```python
from build123d import *

# Parameters (mm, degrees)
SKETCH1_W               = 41.75
SKETCH1_H               = 14
BOSS_EXTRUDE1_DEPTH     = 6.5
SKETCH2_W               = 18
SKETCH2_H               = 14
BOSS_EXTRUDE2_DEPTH     = 26.8
CUT_EXTRUDE1_DEPTH      = 56.20826478
CUT_EXTRUDE1_DEPTH_BACK = 56.20826478
SKETCH3_R               = 4
SKETCH4_R               = 2.75
CUT_EXTRUDE2_DEPTH      = 52.549030059


with BuildPart() as part:
    # Sketch1 → Boss-Extrude1 (new body)
    with BuildSketch(Plane(origin=(0, 0, 0), x_dir=(1, 0, 0), z_dir=(0, 1, 0))):
        with Locations((20.875, 7)):
            Rectangle(SKETCH1_W, SKETCH1_H)
    extrude(amount=BOSS_EXTRUDE1_DEPTH)

    # Sketch2 → Boss-Extrude2 (add)
    with BuildSketch(Plane(origin=(0, 6.5, 0), x_dir=(1, 0, 0), z_dir=(0, 1, 0))):
        with Locations((20.875, 7)):
            Rectangle(SKETCH2_W, SKETCH2_H)
    extrude(amount=BOSS_EXTRUDE2_DEPTH)

    # Sketch3 → Cut-Extrude1 (cut, two sides: drawn at the far end of the back side and taken through both)
    with BuildSketch(Plane.XY.offset(-CUT_EXTRUDE1_DEPTH_BACK)):
        with Locations((20.875, 20)):
            Circle(SKETCH3_R)
    extrude(amount=CUT_EXTRUDE1_DEPTH + CUT_EXTRUDE1_DEPTH_BACK, mode=Mode.SUBTRACT)

    # Sketch4 → Cut-Extrude2 (cut, through all)
    with BuildSketch(Plane(origin=(0, 6.5, 0), x_dir=(1, 0, 0), z_dir=(0, 1, 0))):
        with Locations(Location((37, 7, 0), (0, 0, 270))):
            Circle(SKETCH4_R)
        with Locations(Location((4.75, 7, 0), (0, 0, 270))):
            Circle(SKETCH4_R)
    extrude(amount=-CUT_EXTRUDE2_DEPTH, mode=Mode.SUBTRACT)


solid = part.part
```
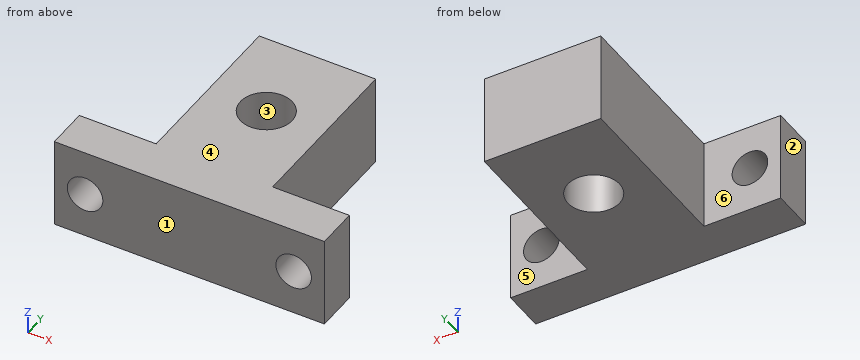
Can you work these out from the model? Positions are in its coordinate system, mm. Face numbers are marked on the shaded views. A direction names the side the tool comes from. Coordinates: 2 decimals unless noted, no trailing zeros. Loops run counter-clockwise (first coordinate to the right, second up) from the corner with the lowest first, then second, coordinate; pieces in that order, holes last.
1) Imagine slicing it at B-B on y = 20. List the corners of the cut face in (x, z) for me (3 decimals).
2) Which directions (+Z, -Z, +X, -X, +Y, -Y) give clear straight access to the entire face, cutting with the end or side of a thin tool? Please do the marked faces 4, 5 and 6.
3) Imagine slicing it at C-C on x = 4.75. List the corners of the cut face in (y, z) for me.
4) I need wall thicknesses on probe 1 along X at (y, z) = (3, -7); probe 2 along X at (y, z) = (20, -6) (3 decimals); probe 3 along Y at (x, z) = (19.5, -12). Which ranges of each line are inside material? Lowest first, please.
5) For pin 1 (6 mm diameter, centred on x = 4, z = -4, fed in from +Y); pin 2 (6 mm diameter, centred on x = 7, y = 20.5, fed in from +Z); pin 3 (6 mm diameter, centred on y = 20, z = -11, fed in from +X) (3 decimals), each with a flat end and sliding along its axis, tell me the tip position at first contact or that it passes through.
6) Imagine slicing it at A-A on z = -7. List the corners of the cut face in (x, y) for me (3 decimals).
7) Thinking about a two-plate mould opening in X: for the marked faces 1, 2 and 3, which applies, pulls with the +X half, pulls with the -X half, needs draft (parallel to the pull), parting line crosses it, or undercut?
8) Imagine slicing it at D-D on z = -1.25. List the corners of the cut face in (x, y) for me (3 decimals), plus the area to 3 significant figures.
Completed:
1. outline: (11.875, -14) - (16.875, -14) - (16.875, 0) - (11.875, 0) - close; (24.875, -14) - (29.875, -14) - (29.875, 0) - (24.875, 0) - close
2. face 4: +Z, +X, -X, +Y, -Y
2. face 5: +Z, -Z, +X, +Y
2. face 6: +Z, -Z, -X, +Y
3. outline: (0, -14) - (6.5, -14) - (6.5, -9.75) - (0, -9.75) - close; (0, -4.25) - (6.5, -4.25) - (6.5, 0) - (0, 0) - close
4. probe 1: x = 0 to 2, 7.5 to 34.25, 39.75 to 41.75
4. probe 2: x = 11.875 to 16.875, 24.875 to 29.875
4. probe 3: y = 0 to 16.24, 23.76 to 33.3
5. pin 1: stops at y = 6.5
5. pin 2: passes through
5. pin 3: stops at x = 29.875
6. outline: (0, 0) - (2, 0) - (2, 6.5) - (0, 6.5) - close; (7.5, 0) - (34.25, 0) - (34.25, 6.5) - (29.875, 6.5) - (29.875, 33.3) - (11.875, 33.3) - (11.875, 6.5) - (7.5, 6.5) - close; (39.75, 0) - (41.75, 0) - (41.75, 6.5) - (39.75, 6.5) - close; hole circle Ø8 at (20.875, 20)
7. face 1: needs draft
7. face 2: pulls with the -X half
7. face 3: undercut
8. outline: (0, 0) - (41.75, 0) - (41.75, 6.5) - (29.875, 6.5) - (29.875, 33.3) - (11.875, 33.3) - (11.875, 6.5) - (0, 6.5) - close; hole circle Ø8 at (20.875, 20)
8. area: 704 mm2
